Job drawing, mm, ordinate dimensions from the low corner. One solid piece. Give positions to 0.01 mm unless a question says otherwise; leave off trailing zeros. Order: outer loops, then holes, each group sorted by start corner. A loop starts at its lowest first (then second) coordinate and runs counter-clockwise, first axis right, second up.
Item 1: Band-saw the part on A-A on y = 46. Give the cut face in (x, z).
Item 2: Wall check: L1, parallel to X at y = 38.5, z = 1.55; L2, parallel to Y at x = 15.5, z = 1.45; L3, parallel to Y at x = 2, z = 0.5. Give the ranges that are in metal, low to high.
Item 3: Flat gauge pins, fed straight in: P1, Ø12, axis at x = 11, y = 31, coming from the +Z side; P2, Ø12, axis at x = 15, y = 36, coming from the +Z side. Where does each tip first touch, or does it go through?
Item 4: Band-saw the part on B-B on x = 26. Give the cut face in (y, z).
Item 5: Band-saw the part on C-C on z = 1.65. Give the cut face in (x, y) (3 decimals), plus the area to 3 significant figures.
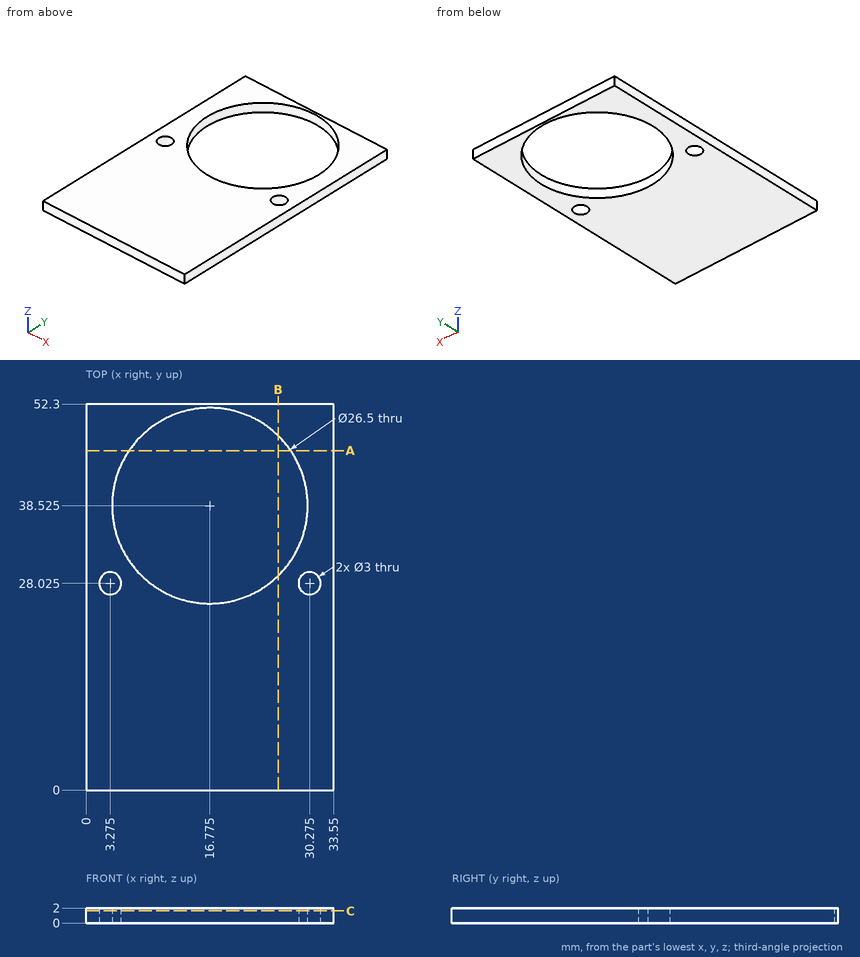
The answers:
1. outline: (0, 0) - (5.83, 0) - (5.83, 2) - (0, 2) - close; (27.72, 0) - (33.55, 0) - (33.55, 2) - (27.72, 2) - close
2. L1: x = 0 to 3.53, 30.02 to 33.55
2. L2: y = 0 to 25.34, 51.71 to 52.3
2. L3: y = 0 to 27.23, 28.82 to 52.3
3. P1: stops at z = 2
3. P2: passes through
4. outline: (0, 0) - (29.01, 0) - (29.01, 2) - (0, 2) - close; (48.04, 0) - (52.3, 0) - (52.3, 2) - (48.04, 2) - close
5. outline: (0, 0) - (33.55, 0) - (33.55, 52.3) - (0, 52.3) - close; hole circle Ø3 at (3.275, 28.025); hole circle Ø26.5 at (16.775, 38.525); hole circle Ø3 at (30.275, 28.025)
5. area: 1,190 mm2
